from build123d import *

# Parameters (mm, degrees)
SKETCH1_R           = 125
BOSS_EXTRUDE1_DEPTH = 20
SKETCH2_R           = 50
CUT_EXTRUDE1_DEPTH  = 20
SKETCH3_R           = 8.132820197
CUT_EXTRUDE2_DEPTH  = 20
SKETCH4_R           = 15
CUT_EXTRUDE3_DEPTH  = 10
SKETCH5_R           = 7.5
CUT_EXTRUDE4_DEPTH  = 10
CIRPATTERN1_COUNT   = 4


with BuildPart() as part:
    # Sketch1 → Boss-Extrude1 (new body)
    with BuildSketch(Plane.XY):
        Circle(SKETCH1_R)
    extrude(amount=BOSS_EXTRUDE1_DEPTH)

    # Sketch2 → Cut-Extrude1 (cut)
    with BuildSketch(Plane.XY.offset(20)):
        Circle(SKETCH2_R)
    extrude(amount=-CUT_EXTRUDE1_DEPTH, mode=Mode.SUBTRACT)

    # Sketch3 → Cut-Extrude2 (cut)
    with BuildSketch(Plane.XY.offset(20)):
        with Locations((0, 107.5)):
            Circle(SKETCH3_R)
    cut_extrude2 = extrude(amount=-CUT_EXTRUDE2_DEPTH, mode=Mode.SUBTRACT)

    # Sketch4 → Cut-Extrude3 (cut)
    with BuildSketch(Plane(origin=(0, 0, 0), x_dir=(-1, 0, 0), z_dir=(0, 0, -1))):
        with Locations((49.497474683, 49.497474683)):
            Circle(SKETCH4_R)
    cut_extrude3 = extrude(amount=-CUT_EXTRUDE3_DEPTH, mode=Mode.SUBTRACT)

    # Sketch5 → Cut-Extrude4 (cut)
    with BuildSketch(Plane(origin=(0, 0, 10), x_dir=(-1, 0, 0), z_dir=(0, 0, -1))):
        with Locations((49.497474683, 49.497474683)):
            Circle(SKETCH5_R)
    cut_extrude4 = extrude(amount=-CUT_EXTRUDE4_DEPTH, mode=Mode.SUBTRACT)

    # CirPattern1: Cut-Extrude2, Cut-Extrude3, Cut-Extrude4 ×4 about axis
    cirpattern1_axis = Axis((0, 0, 0), (0, 0, 1))
    add([cut_extrude2.rotate(cirpattern1_axis, i * 360 / CIRPATTERN1_COUNT) for i in range(1, CIRPATTERN1_COUNT)], mode=Mode.SUBTRACT)
    add([cut_extrude3.rotate(cirpattern1_axis, i * 360 / CIRPATTERN1_COUNT) for i in range(1, CIRPATTERN1_COUNT)], mode=Mode.SUBTRACT)
    add([cut_extrude4.rotate(cirpattern1_axis, i * 360 / CIRPATTERN1_COUNT) for i in range(1, CIRPATTERN1_COUNT)], mode=Mode.SUBTRACT)


solid = part.part
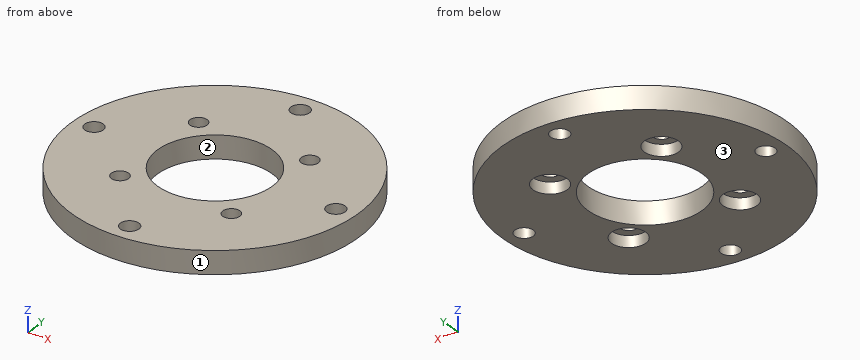
Input: part model. Units: mm. Frame: model coordinates. Face numbers are marked on the shaded views. Give positions to 0.01 mm unless a question says otherwise; leave off trailing zeros. Loops run counter-clockwise (first coordinate to the right, second up) from the corner with the lowest first, then second, coordinate; pieces in that order, holes last. Notation, with made-up numbers: (13, -24) - (31, -24) arc R33 cw to (31, 15) - close; hole circle Ø5 at (85, -7). An arc over 180 degrees is marked (long way). Use CSV: the item, a comma, the result in double quotes. Start each with the question number.
Item 1: Section A-A on y = 0. Return loops of the section in (x, z).
Item 2: Section C-C on y = -107.5. Return loops of the section in (x, z).
Item 3: Mould query, pull axis X, two halves, no side actions, for the marked faces 1, 2 and 3. Classes: pulls with the +X half, pulls with the -X half, needs draft (parallel to the pull), parting line crosses it, or undercut.
Item 4: Line query: line 1 (Y direction, x = 0, z = 10.5); line 2 (Y direction, x = -3, z = 10.75); line 3 (X direction, y = 54.5, z = 15). Output: solid intervals per line, ascending.
Item 5: Section D-D on z = 13. State how many separate pieces and enclosed holes the cut face has, then the cut area to 3 significant figures.
Item 6: Contact query for flat-ended pins moving along their axis: P1, Ø9, axis at x = -49.5, y = -49.5, coming from the +Z side; P2, Ø8, axis at y = 25, z = 15.5, coming from the +X side; P3, Ø2, axis at y = 7.5, z = 10, coming from the +X side; P4, Ø15, axis at x = -54, y = 51, coming from the -Z side. Output: stop coordinate, or through.
Ans:
1,outline,"(-125, 0) - (-115.63, 0) - (-115.63, 20) - (-125, 20) - close; (-99.37, 0) - (-50, 0) - (-50, 20) - (-99.37, 20) - close; (50, 0) - (99.37, 0) - (99.37, 20) - (50, 20) - close; (115.63, 0) - (125, 0) - (125, 20) - (115.63, 20) - close"
2,outline,"(-63.79, 0) - (-8.13, 0) - (-8.13, 20) - (-63.79, 20) - close; (8.13, 0) - (63.79, 0) - (63.79, 20) - (8.13, 20) - close"
3,face 1,"parting line crosses it"
3,face 2,"undercut"
3,face 3,"needs draft"
4,line 1,"y = -125 to -115.63, -99.37 to -50, 50 to 99.37, 115.63 to 125"
4,line 2,"y = -124.96 to -115.06, -99.94 to -49.91, 49.91 to 99.94, 115.06 to 124.96"
4,line 3,"x = -112.49 to -55.09, -43.91 to 43.91, 55.09 to 112.49"
5,separate pieces,"1"
5,enclosed holes,"9"
5,area,"39,700 mm2"
6,P1,"passes through"
6,P2,"stops at x = 123.22"
6,P3,"stops at x = 124.83"
6,P4,"stops at z = 10"
